Design review of the part built by this model. Coordinates are the model's own, in mm. Face numbers are marked on the shaded views. A direction names the side the tool comes from. Give positions to 0.01 mm unless a question says otherwise; leave off trailing zeros. Loops run counter-clockwise (first coordinate to the right, second up) from the corner with the lowest first, then second, coordinate; pieces in that order, holes last. Notation, with made-up numbers: (-8, -2.5) -> (14, -2.5) arc R21 ccw to (14, 16.5) -> close; hole circle Ø7 at (86, 33). An arc over 180 degrees is marked (long way). Answer in a Markdown table with one row per item. Add a question column.
(1) Consider section B-B on x = 0. Write out the cut boundary in (y, z), then the cut area to 3 significant figures.
(2) For pin 1 (3 mm diameter, centred on y = -10, z = 17.5, fed in from -X); pin 2 (12 mm diameter, centred on x = -10, y = -17, fed in from -Z); pin 3 (4 mm diameter, centred on x = -32, y = -17, fed in from -Z); pin 4 (6 mm diameter, centred on x = 14.5, y = -6, fed in from +Z), all flat-tipped, find the tip position at first contact; note any pin that passes through.
(3) Consider section D-D on x = -32. Write out the cut boundary in (y, z).
(4) For the marked faces 4, 5 and 6, list the 3-axis set-ups (+Z, -Z, +X, -X, +Y, -Y) from which the entire face can be reached by the end or side of a thin tool; tool diameter is ignored.
(5) For line 1 (Z direction, x = -22, y = -9.75); line 2 (Z direction, x = -0.5, y = -10.75) (3 decimals); line 3 (X direction, y = -12.75, z = 5), list the stretches that pass through material, from the lowest coordinate up.
(6) Consider section A-A on y = -15. Write out the cut boundary in (x, z), then the cut area to 3 significant figures.
(7) Draft analysis for pull direction Y (two halves, no side actions). For the marked faces 1, 2 and 3, state which applies: +Y half, -Y half, draft (parallel to the pull), parting line (faces both ways), or undercut.
(8) Consider section C-C on y = -4.5. Write out the cut boundary in (x, z).
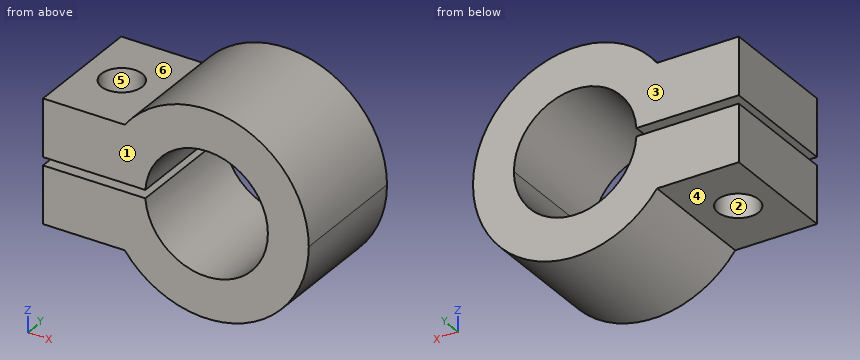
from build123d import *

# Parameters (mm, degrees)
F1_DEPTH = 30
F2_R     = 5
F3_DEPTH = 40.001


with BuildPart() as f1:
    # F0 (on Front) → F1 (new body)
    with BuildSketch(Plane.XZ):
        with BuildLine():
            Line((-40, 1), (-24.9799919936, 1))
            ThreePointArc((-24.9799919936, 1), (-23.5541911331, 8.3785488042), (-20, 15))
            Line((-20, 15), (-40, 15))
            Line((-40, 15), (-40, 1))
        make_face()
        with BuildLine():
            ThreePointArc((-14.9666295471, 1), (0.5002783193, 14.9916550655), (15, 0))
            ThreePointArc((15, 0), (0.5002783193, -14.9916550655), (-14.9666295471, -1))
            Line((-14.9666295471, -1), (-24.9799919936, -1))
            ThreePointArc((-24.9799919936, -1), (-23.5541911331, -8.3785488042), (-20, -15))
            ThreePointArc((-20, -15), (7.9056941504, -23.7170824513), (25, 0))
            ThreePointArc((25, 0), (7.9056941504, 23.7170824513), (-20, 15))
            ThreePointArc((-20, 15), (-23.5541911331, 8.3785488042), (-24.9799919936, 1))
            Line((-24.9799919936, 1), (-14.9666295471, 1))
        make_face()
        with BuildLine():
            ThreePointArc((-20, -15), (-23.5541911331, -8.3785488042), (-24.9799919936, -1))
            Line((-24.9799919936, -1), (-40, -1))
            Line((-40, -1), (-40, -15))
            Line((-40, -15), (-20, -15))
        make_face()
    extrude(amount=F1_DEPTH)

    # F2 (on face) → F3 (cut, through all)
    with BuildSketch(Plane.XY.offset(15)):
        with Locations((-30.2969049662, -15)):
            Circle(F2_R)
    extrude(amount=-F3_DEPTH, mode=Mode.SUBTRACT)


solid = f1.part
Values follow:
| question | item | result |
|---|---|---|
| 1 | outline | (-30, -25) -> (0, -25) -> (0, -15) -> (-30, -15) -> close; (-30, 15) -> (0, 15) -> (0, 25) -> (-30, 25) -> close |
| 1 | area | 600 mm2 |
| 2 | pin 1 | x = -19.21 |
| 2 | pin 2 | z = -24.68 |
| 2 | pin 3 | through |
| 2 | pin 4 | z = 22.2 |
| 3 | outline | (-30, -15) -> (-19.7, -15) -> (-19.7, -1) -> (-30, -1) -> close; (-30, 1) -> (-19.7, 1) -> (-19.7, 15) -> (-30, 15) -> close; (-10.3, -15) -> (0, -15) -> (0, -1) -> (-10.3, -1) -> close; (-10.3, 1) -> (0, 1) -> (0, 15) -> (-10.3, 15) -> close |
| 4 | face 4 | -Z, -X, +Y, -Y |
| 4 | face 5 | +Z, -Z |
| 4 | face 6 | +Z, -X, +Y, -Y |
| 5 | line 1 | -15 to -1, 1 to 15 |
| 5 | line 2 | -24.995 to -14.992, 14.992 to 24.995 |
| 5 | line 3 | -40 to -34.76, -25.83 to -14.14, 14.14 to 24.49 |
| 6 | outline | (-40, -15) -> (-35.3, -15) -> (-35.3, -1) -> (-40, -1) -> close; (-40, 1) -> (-35.3, 1) -> (-35.3, 15) -> (-40, 15) -> close; (-25.3, -15) -> (-20, -15) arc R25 ccw (long way) to (-20, 15) -> (-25.3, 15) -> (-25.3, 1) -> (-14.97, 1) arc R15 cw (long way) to (-14.97, -1) -> (-25.3, -1) -> close |
| 6 | area | 1,420 mm2 |
| 7 | face 1 | -Y half |
| 7 | face 2 | undercut |
| 7 | face 3 | +Y half |
| 8 | outline | (-40, -15) -> (-20, -15) arc R25 ccw (long way) to (-20, 15) -> (-40, 15) -> (-40, 1) -> (-14.97, 1) arc R15 cw (long way) to (-14.97, -1) -> (-40, -1) -> close |
